The listing builds one solid part. Answer for the finished solid, in the listing's coordinates (mm). Round coordinates to 2 decimals unless told otherwise and drop trailing zeros. Write each loop counter-clockwise with the first axis right and the second up, starting at its lowest first coordinate (ties: lowest second). Pieces come first, ordered by that corner, then holes. Notation, with made-up numbers: (64, -19) - (94, -19) arc R28 cw to (94, 6) - close; hole circle Ø10 at (42, 87.25). An arc over 180 degrees is marked (long way). Answer in a Markdown table with one row per item.
Autodesk Inventor part; units mm, degrees
ref_plane "Work Plane1" through (0, 76.2, 0) normal (0, 1, 0) x (-1, 0, 0)
ref_plane "YZ Plane" through (0, 0, 0) normal (1, 0, 0) x (0, 1, 0)
ref_plane "XY Plane" through (0, 0, 0) normal (0, 0, 1) x (1, 0, 0)
sketch "Sketch2" plane through (0, 0, 0) normal (1, 0, 0) x (0, 1, 0)
  line L0 (0, 0) -> (76.2, 0) construction
  line L1 (0, 0) -> (0, -76.2) construction
  line L2 (0, 0) -> (0, 76.2) construction
  line L3 (76.2, 0) -> (0, 76.2)
  dimension "d0" = 76.2
  dimension "d1" = 76.2
  dimension "d2" = 76.2
sketch "Sketch3" plane through (0, 0, 0) normal (0, 0, 1) x (1, 0, 0)
  line L0 (0, 0) -> (0, 76.2) construction
  line L1 (0, 0) -> (-76.2, 0) construction
  line L2 (0, 76.2) -> (-76.2, 0)
  dimension "d3" = 76.2
  dimension "d4" = 76.2
ref_plane "Work Plane1" through (0, 76.2, 0) normal (0, 1, 0) x (-1, 0, 0)
sketch "Sketch4" plane through (0, 76.2, 0) normal (0, 1, 0) x (-1, 0, 0)
  circle A0 centre (0, 0) radius 12.7
  dimension "d6" = 25.4
sweep "Sweep1" add profiles "Sketch4" path "Sketch3"
sketch "Sketch5" plane through (0, 76.2, 0) normal (0, 1, 0) x (-1, 0, 0)
  circle A0 centre (0, 0) radius 12.7
sweep "Sweep3" add profiles "Sketch5" path "Sketch2"
sketch "Sketch6" plane through (0, 0, 0) normal (1, 0, 0) x (0, 1, 0)
  line L0 (76.2, 8.9803) -> (76.2, -12.7)
  line L1 (76.2, 0) -> (0, -76.2)
  point P0 (0, 0)
  point P1 (76.2, -8.9803)
  dimension "d13" = 76.2
sketch "Sketch7" plane through (0, 76.2, 0) normal (0, 1, 0) x (-1, 0, 0)
  circle A0 centre (0, 0) radius 12.7
sweep "Sweep4" add profiles "Sketch7" path "Sketch6" path curves L1
sketch "Sketch10" plane through (0, 0, 0) normal (0, 1, 0) x (-1, 0, 0)
  circle A0 centre (0, 76.2) radius 12.7
  circle A1 centre (0, -76.2) radius 12.7
  circle A2 centre (76.2, 0) radius 12.7
  line L0 (-12.7, 76.2) -> (-12.7, -76.2)
  line L1 (6.7517, -86.9566) -> (86.5852, -7.3102)
  circle A3 centre (76.2, 0) radius 12.7
  line L2 (84.8484, 9.3002) -> (8.981, 85.1796)
  point P0 (0, 0)
extrude "Extrusion1" add sketch "Sketch10" against normal blind 12.7 contours A0 | A0 L2 A2 L1 A1 L0 | A2 L1 | A1 L1 picked at (77.9931, 4.4447) picked at (3.5769, -74.7711)
properties part number "CameraTripodBaseV02"
(1) Section A-A (y = -5.5) is taken. Give the vertices of the cut face in (x, z), and give its area (3 significant figures).
Checked values:
| item | result |
|---|---|
| outline | (-86.59, -7.31) - (-6.75, -86.96) arc R12.7 ccw to (12.7, -76.2) - (12.7, 76.2) arc R12.7 ccw to (-8.98, 85.18) - (-84.85, 9.3) arc R12.7 ccw to start |
| area | 11,000 mm2 |
(2) Flat-ended cylindrical pins translate along their axes: pin 1 (10 mm diameter, centred on y = 52, z = -29.5, fed in from -X); pin 2 (4 mm diameter, centred on x = -49.5, y = 29, fed in from +Z); pin 3 (8 mm diameter, centred on x = -26.5, z = 24.5, fed in from +Y). Find the tip coordinate at first contact, or state that the pin passes through.
Checked values:
| item | result |
|---|---|
| pin 1 | stops at x = -12.7 |
| pin 2 | stops at z = 12.7 |
| pin 3 | stops at y = 0 |
(3) Find the intervals of material crossed by line 1 (Z direction, x = 2, y = 59.5); line 2 (Z direction, x = -11.5, y = 25.5); line 3 (Y direction, x = -46, z = 41.5), in increasing order.
Checked values:
| item | result |
|---|---|
| line 1 | z = -29.24 to -4.16, 4.16 to 29.24 |
| line 2 | z = -56.09 to -45.31, 45.31 to 56.09 |
| line 3 | y = -12.7 to 0 |
(4) For a pull along Y with two mould halves and no side action, classify faces 1 (the flat face through (-26, -12.7, 1)), 2 (the flat face through (-25, 0, 2)), 3 (the flat face through (0, 76.2, 0)), 4 (the cylindrical face through (6.31, -6.26, -87.22)) as pulls with the +Y half, pulls with the -Y half, needs draft (parallel to the pull), parting line crosses it, or undercut.
Checked values:
| item | result |
|---|---|
| face 1 | pulls with the -Y half |
| face 2 | undercut |
| face 3 | pulls with the +Y half |
| face 4 | needs draft |
(5) Section B-B (y = 30) is taken. State how many separate pieces and enclosed holes the cut face has, and give its area (3 significant figures).
Checked values:
| item | result |
|---|---|
| separate pieces | 3 |
| enclosed holes | 0 |
| area | 1,520 mm2 |
